Geometry check sheet. Reference: the model listing, model coordinates, mm. A direction names the side the tool comes from. Give positions to 0.01 mm unless a question says otherwise; leave off trailing zeros. Order: outer loops, then holes, each group sorted by start corner. A loop starts at its lowest first (then second) coordinate and runs counter-clockwise, first axis right, second up. Notation, with made-up numbers: M -4.75,60.5 L 26.25,60.5 A23 ccw 26.25,96.5 Z; hole C 30,35.5 d4. An arc over 180 degrees is marked long. Answer as CSV lines item,"result". Start each with the question number.
```python
from build123d import *

# Parameters (mm, degrees)
F0_R     = 27.0435400324
F1_DEPTH = 25.4
F3_D     = 38.1
F5_DEPTH = 25.4
F6_DEPTH = 127


with BuildPart() as f1:
    # F0 (on Front) → F1 (new body)
    with BuildSketch(Plane.XZ):
        with Locations((27.6412703097, 27.8783403337)):
            Circle(F0_R)
    extrude(amount=F1_DEPTH)

    # F3 (through all)
    with Locations(Plane.XZ.offset(25.4)):
        with Locations((27.6412703097, 27.8783403337)):
            Hole(F3_D / 2)

    # F4 (on face) → F5 (cut)
    with BuildSketch(Plane(origin=(0, 0, 0), x_dir=(-1, 0, 0), z_dir=(0, 1, 0))):
        with BuildLine():
            Line((-26.2493573993, 5.0403885543), (-26.2493573993, 8.8792593441))
            ThreePointArc((-26.2493573993, 8.8792593441), (-27.6329506683, 8.8283421504), (-29.0165878832, 8.8780508209))
            Line((-29.0165878832, 8.8780508209), (-29.0165878832, 5.0403885543))
            Line((-29.0165878832, 5.0403885543), (-26.2493573993, 5.0403885543))
        make_face()
    extrude(amount=-F5_DEPTH, mode=Mode.SUBTRACT)

    # F6 (add): a face of the model
    f6_faces = [f1.faces().sort_by_distance(p)[0] for p in [
        (1.362637099, -25.4, 27.8783403337),
    ]]
    extrude(f6_faces, amount=F6_DEPTH)


solid = f1.part
```
Item 1: Section check D-D on x = 49. Record the boundary of the cut face in (y, z).
Item 2: Access from +Z, -Z, +X, -X, +Y, -Y to the whole of each face (thin tool, end or side, straight path). Record for faces 1 (the face through (26.249, -75, 7)), 2 (the face through (9, 0, 22)).
Item 3: Section check C-C on z = 40.5. Record the boundary of the cut face in (x, y), then the cut area to 3 significant figures.
Item 4: Section check A-A on y = -101. Record the boundary of the cut face in (x, z).
Item 5: Scan lines: line 1 along X through (y, z) = (-88, 28); line 2 along Z through (x, y) = (21.5, -60); line 3 along X through (y, z) = (-31, 45). Record each from-to range of solid material in increasing order.
Item 6: Draft check along X on faces 3 (the face through (42.18, -75.13, 50.68)), 4 (the face through (28, -75, 5.04)), 5 (the face through (29.017, -75, 7)), 6 (the face through (9, -152.4, 22)). Enter one of: pulls with the +X half, pulls with the -X half, needs draft (parallel to the pull), parting line crosses it, or undercut.
Item 7: Section check B-B on x = 18.5. Record the boundary of the cut face in (y, z).
Item 8: Depth check by flat-ended pin: pin 1 Ø1 at (y, z) = (-107, 33.5) entering from -X; pin 2 Ø1.4 at (x, y) = (27, -80.5) entering from +Z; pin 3 Ø1.2 at (y, z) = (-92, 7.5) entering from -X. Enter the tip coordinate at first touch or a pass-through.
Numbers:
1,outline,"M -152.4,11.29 L 0,11.29 L 0,44.47 L -152.4,44.47 Z"
2,face 1,"+Y, -Y"
2,face 2,"+Z, -Z, +X, -X, +Y"
3,outline,"M 3.72,-152.4 L 13.37,-152.4 L 13.37,0 L 3.72,0 Z; M 41.91,-152.4 L 51.56,-152.4 L 51.56,0 L 41.91,0 Z"
3,area,"2,940 mm2"
4,outline,"C 27.64,27.88 d54.09; hole M 26.25,5.04 L 29.02,5.04 L 29.02,8.88 A19.05 ccw long 26.25,8.88 Z"
5,line 1,"0.6 to 8.59, 46.69 to 54.68"
5,line 2,"1.54 to 9.85, 45.91 to 54.22"
5,line 3,"6.71 to 19.29, 35.99 to 48.57"
6,face 3,"parting line crosses it"
6,face 4,"undercut"
6,face 5,"undercut"
6,face 6,"needs draft"
7,outline,"M -152.4,2.43 L 0,2.43 L 0,11.16 L -152.4,11.16 Z; M -152.4,44.59 L 0,44.59 L 0,53.33 L -152.4,53.33 Z"
8,pin 1,"x = 1.09"
8,pin 2,"z = 54.92"
8,pin 3,"x = 9.2"
